The listing builds one solid part. Answer for the finished solid, in the listing's coordinates (mm). A direction names the side the tool comes from. Give positions to 0.01 mm unless a question says otherwise; leave off trailing zeros. Write each loop counter-clockwise with the first axis right and the second up, starting at its lowest first coordinate (ties: lowest second). Pieces come first, ordered by that corner, then holes. Notation, with made-up numbers: (29, 57) -> (44, 57) arc R27 ccw to (44, 85) -> close; hole circle Ø3 at (56, 72.5). An arc over 180 degrees is marked (long way). One line per question, with ' | ' between items.
from build123d import *

# Parameters (mm, degrees)
SKETCH1_R           = 75
BOSS_EXTRUDE1_DEPTH = 20
SKETCH2_R           = 60
BOSS_EXTRUDE2_DEPTH = 10
SKETCH3_R           = 75
BOSS_EXTRUDE3_DEPTH = 20
SKETCH4_R           = 30
BOSS_EXTRUDE4_DEPTH = 100
SKETCH5_R           = 100
BOSS_EXTRUDE5_DEPTH = 150
SKETCH6_R           = 80
BOSS_EXTRUDE6_DEPTH = 70


with BuildPart() as part:
    # Sketch1 → Boss-Extrude1 (new body)
    with BuildSketch(Plane(origin=(0, 0, 0), x_dir=(1, 0, 0), z_dir=(0, 1, 0))):
        with Locations(Location((0, 0, 0), (0, 0, 270))):
            Circle(SKETCH1_R)
    extrude(amount=BOSS_EXTRUDE1_DEPTH)

    # Sketch2 → Boss-Extrude2 (add)
    with BuildSketch(Plane(origin=(0, 20, 0), x_dir=(1, 0, 0), z_dir=(0, 1, 0))):
        with Locations(Location((0, 0, 0), (0, 0, 270))):
            Circle(SKETCH2_R)
    extrude(amount=BOSS_EXTRUDE2_DEPTH)

    # Sketch3 → Boss-Extrude3 (add)
    with BuildSketch(Plane(origin=(0, 30, 0), x_dir=(1, 0, 0), z_dir=(0, 1, 0))):
        with Locations(Location((0, 0, 0), (0, 0, 270))):
            Circle(SKETCH3_R)
    extrude(amount=BOSS_EXTRUDE3_DEPTH)

    # Sketch4 → Boss-Extrude4 (add)
    with BuildSketch(Plane(origin=(0, 50, 0), x_dir=(1, 0, 0), z_dir=(0, 1, 0))):
        with Locations(Location((0, 0, 0), (0, 0, 270))):
            Circle(SKETCH4_R)
    extrude(amount=BOSS_EXTRUDE4_DEPTH)

    # Sketch5 → Boss-Extrude5 (add)
    with BuildSketch(Plane(origin=(0, 0, 0), x_dir=(0, 0, -1), z_dir=(1, 0, 0))):
        with Locations((0, 154.201763101)):
            Circle(SKETCH5_R)
    extrude(amount=-BOSS_EXTRUDE5_DEPTH)

    # Sketch6 → Boss-Extrude6 (add)
    with BuildSketch(Plane(origin=(0, 0, 0), x_dir=(0, 0, -1), z_dir=(1, 0, 0))):
        with Locations(Location((0, 154.201763101, 0), (0, 0, 247.975687163))):
            Circle(SKETCH6_R)
    extrude(amount=BOSS_EXTRUDE6_DEPTH)


solid = part.part
Item 1: Find section C-C (y = 146). Write down the section's boundary in (x, z), then the cut area to 3 significant figures.
Answers below:
outline: (-150, -99.66) -> (0, -99.66) -> (0, -79.58) -> (70, -79.58) -> (70, 79.58) -> (0, 79.58) -> (0, 99.66) -> (-150, 99.66) -> close | area: 41,000 mm²
Item 2: Find section B-B (z = 67). Write down the section's boundary in (x, y), then the cut area to 3 significant figures.
Answers below:
outline: (-150, 79.97) -> (0, 79.97) -> (0, 110.49) -> (70, 110.49) -> (70, 197.92) -> (0, 197.92) -> (0, 228.44) -> (-150, 228.44) -> close; (-33.7, 0) -> (33.7, 0) -> (33.7, 20) -> (-33.7, 20) -> close; (-33.7, 30) -> (33.7, 30) -> (33.7, 50) -> (-33.7, 50) -> close | area: 31,100 mm²
Item 3: Consider line 1 (X direction, y = 144, z = -15.5); line 2 (X direction, y = 134, z = -83); line 3 (Z direction, x = -121, y = 151). Determine where each line is inside the solid, lowest interval first. Write a range as [from, to].
Answers below:
line 1: [-150, 70] | line 2: [-150, 0] | line 3: [-99.95, 99.95]
Item 4: Flat-ended cylindrical pins translate along their axes: pin 1 (10 mm diameter, centred on x = -125, z = 69, fed in from -Y); pin 2 (12 mm diameter, centred on x = -97, y = 179, fed in from +Z); pin 3 (4 mm diameter, centred on x = -14, y = 56, fed in from +Z). Find the tip coordinate at first contact, or state that the pin passes through.
Answers below:
pin 1: y = 77.36 | pin 2: z = 98.22 | pin 3: z = 27.5
Item 5: A tool of negligible diameter and unlimited length cuts with its end or side. For faces 1 (the face through (0, 229, 30)), 2 (the face through (2.64, 24.93, -59.94)), 3 (the face through (70, 155, -1)), 4 (the face through (-45.636, 9.86, -59.517)), 5 (the face through (-150, 156, 1)), from which of +Z, -Z, +X, -X, +Y, -Y can it reach the whole face along a straight path? Write none if from no direction.
Answers below:
face 1: +X | face 2: none | face 3: +Z, -Z, +X, +Y | face 4: -Y | face 5: +Z, -Z, -X, +Y, -Y
Item 6: Find section D-D (x = 11). Write down the section's boundary in (y, z), then the cut area to 3 significant figures.
Answers below:
outline: (0, -74.19) -> (20, -74.19) -> (20, -58.98) -> (30, -58.98) -> (30, -74.19) -> (50, -74.19) -> (50, -27.91) -> (79.23, -27.91) arc R80 ccw (long way) to (79.23, 27.91) -> (50, 27.91) -> (50, 74.19) -> (30, 74.19) -> (30, 58.98) -> (20, 58.98) -> (20, 74.19) -> (0, 74.19) -> close | area: 28,700 mm²
Item 7: Determine the mould class of faces 6 (the face through (50, 20, -34)), 7 (the face through (1, 0, -1)), 8 (the face through (-45.636, 39.86, -59.517)) for opening direction Y: pulls with the +Y half, pulls with the -Y half, needs draft (parallel to the pull), parting line crosses it, or undercut.
Answers below:
face 6: undercut | face 7: pulls with the -Y half | face 8: needs draft
Item 8: Find section A-A (z = 0). Write down the section's boundary in (x, y), then the cut area to 3 significant figures.
Answers below:
outline: (-150, 54.2) -> (-30, 54.2) -> (-30, 50) -> (-75, 50) -> (-75, 30) -> (-60, 30) -> (-60, 20) -> (-75, 20) -> (-75, 0) -> (75, 0) -> (75, 20) -> (60, 20) -> (60, 30) -> (75, 30) -> (75, 50) -> (30, 50) -> (30, 74.2) -> (70, 74.2) -> (70, 234.2) -> (0, 234.2) -> (0, 254.2) -> (-150, 254.2) -> close | area: 49,300 mm²
